Autodesk Inventor part; units mm, degrees
ref_plane "Start plane" through (0, 0, 0) normal (0, 0, 1) x (1, 0, 0)
ref_plane "End plane" through (0, 0, 500) normal (0, 0, 1) x (1, 0, 0)
ref_plane "YZ Plane" through (0, 0, 0) normal (1, 0, 0) x (0, 1, 0)
ref_plane "Start plane" through (0, 0, 0) normal (0, 0, 1) x (1, 0, 0)
ref_plane "End plane" through (0, 0, 500) normal (0, 0, 1) x (1, 0, 0)
sketch "Sketch" plane through (0, 0, 0) normal (0, 0, 1) x (1, 0, 0)
  line L0 (-9.2, 25) -> (9.2, 25)
  line L1 (15, 19.2) -> (15, -19.2)
  line L2 (9.2, -25) -> (-9.2, -25)
  line L3 (-15, -19.2) -> (-15, 19.2)
  arc A0 (-9.2, 25) -> (-15, 19.2) centre (-9.2, 19.2) ccw
  arc A1 (15, 19.2) -> (9.2, 25) centre (9.2, 19.2) ccw
  arc A2 (9.2, -25) -> (15, -19.2) centre (9.2, -19.2) ccw
  arc A3 (-15, -19.2) -> (-9.2, -25) centre (-9.2, -19.2) ccw
  line L4 (-22.6817, 0) -> (22.6817, 0) construction
  line L5 (0, -36.6817) -> (0, 36.6817) construction
  arc A4 (-9.2, 22.1) -> (-12.1, 19.2) centre (-9.2, 19.2) ccw
  line L6 (-9.2, 22.1) -> (9.2, 22.1)
  arc A5 (12.1, 19.2) -> (9.2, 22.1) centre (9.2, 19.2) ccw
  line L7 (12.1, 19.2) -> (12.1, -19.2)
  arc A6 (9.2, -22.1) -> (12.1, -19.2) centre (9.2, -19.2) ccw
  line L8 (9.2, -22.1) -> (-9.2, -22.1)
  arc A7 (-12.1, -19.2) -> (-9.2, -22.1) centre (-9.2, -19.2) ccw
  line L9 (-12.1, -19.2) -> (-12.1, 19.2)
  point P0 (-15, 25)
  point P1 (15, -25)
  point P2 (15, 25)
  dimension "b" = 30
  dimension "ParH" = 50
  dimension "msp_r" = 5.8
  dimension "d8" = 15
  dimension "d9" = 25
  dimension "d10" = 2.9
extrude "Body" add sketch "Sketch" along normal up to surface (500 mm away) from surface at 0
sketch "Sketch2" plane through (0, 0, 0) normal (0, 0, 1) x (1, 0, 0)
  line L0 (0, 0) -> (10, 0)
ref_plane "Work Plane3" through (0, 0, 0) normal (0, -1, 0) x (1, 0, 0)
sketch "Sketch3" plane through (0, 0, 0) normal (0, -1, 0) x (1, 0, 0)
  line L0 (-2, 0) -> (12, 0)
  line L1 (-2, 500) -> (12, 500)
  dimension "d14" = 500
equation "\"msp_r\" = 2 * ParT"
equation "\"d8\" = 0.5 * b"
equation "\"d9\" = 0.5 * ParH"
equation "\"d10\" = ParT"
equation "\"G_OFFSET_START\" = 0"
equation "\"G_OFFSET_END\" = 0"
equation "\"G_L\" = d14"
properties part number "DIN 59 410 - 50x30x2.9-500" material "Steel, Mild, Welded"
Design review of the part built by this model. Coordinates are the model's own, in mm. A direction names the side the tool comes from. Coordinates: 2 decimals unless noted, no trailing zeros. Write each loop counter-clockwise with the first axis right and the second up, starting at its lowest first coordinate (ties: lowest second). Pieces come first, ordered by that corner, then holes.
1) Add section C-C (z = 321.5). Write out the cut boundary in (x, y).
2) Mouldability with a two-part tool opening along X and no side actions: class faces 3 (the flat face through (-12.3, 2, 500)), 4 (the flat face through (15, 0, 246)), 5 (the flat face through (-12.1, 0, 246)) as +X half, -X half, draft (parallel to the pull), parting line (faces both ways), or undercut.
3) To check wall thickness, follow L1, parallel to X at y = 16, z = 173.5; L2, parallel to Y at x = -9.25, z = 363.5; L3, parallel to X at y = -21, z = 223.5. State the ranges of each line that lie inside material, in increasing order.
4) Add section A-A (y = -11). Write out the cut boundary in (x, z), plus the area to 3 significant figures.
5) Insertion check: pin 1 (3 mm diameter, centred on y = 20, z = 342, fed in from +X). The pin has a flat end and moves straight along its axis. Give the tip position at first contact, or say it passes through.
6) Machinability: for faces 1 (the flat face through (12.1, 0, 246)), 2 (the flat face through (-12.3, 2, 0)), which of the approach directions +Z, -Z, +X, -X, +Y, -Y give a long, thin tool a straight path to every point of the face, cutting with its end or side? Answer none if there is none.
7) Add section B-B (x = 5). Write out the cut boundary in (y, z).
Check result:
1. outline: (-15, -19.2) arc R5.8 ccw to (-9.2, -25) - (9.2, -25) arc R5.8 ccw to (15, -19.2) - (15, 19.2) arc R5.8 ccw to (9.2, 25) - (-9.2, 25) arc R5.8 ccw to (-15, 19.2) - close; hole (-12.1, -19.2) arc R2.9 ccw to (-9.2, -22.1) - (9.2, -22.1) arc R2.9 ccw to (12.1, -19.2) - (12.1, 19.2) arc R2.9 ccw to (9.2, 22.1) - (-9.2, 22.1) arc R2.9 ccw to (-12.1, 19.2) - close
2. face 3: draft
2. face 4: +X half
2. face 5: undercut
3. L1: x = -15 to -12.1, 12.1 to 15
3. L2: y = -25 to -22.1, 22.1 to 25
3. L3: x = -14.71 to -11.47, 11.47 to 14.71
4. outline: (-15, 0) - (-12.1, 0) - (-12.1, 500) - (-15, 500) - close; (12.1, 0) - (15, 0) - (15, 500) - (12.1, 500) - close
4. area: 2,900 mm2
5. pin 1: stops at x = 15
6. face 1: +Z, -Z
6. face 2: -Z, +X, -X, +Y, -Y
7. outline: (-25, 0) - (-22.1, 0) - (-22.1, 500) - (-25, 500) - close; (22.1, 0) - (25, 0) - (25, 500) - (22.1, 500) - close
